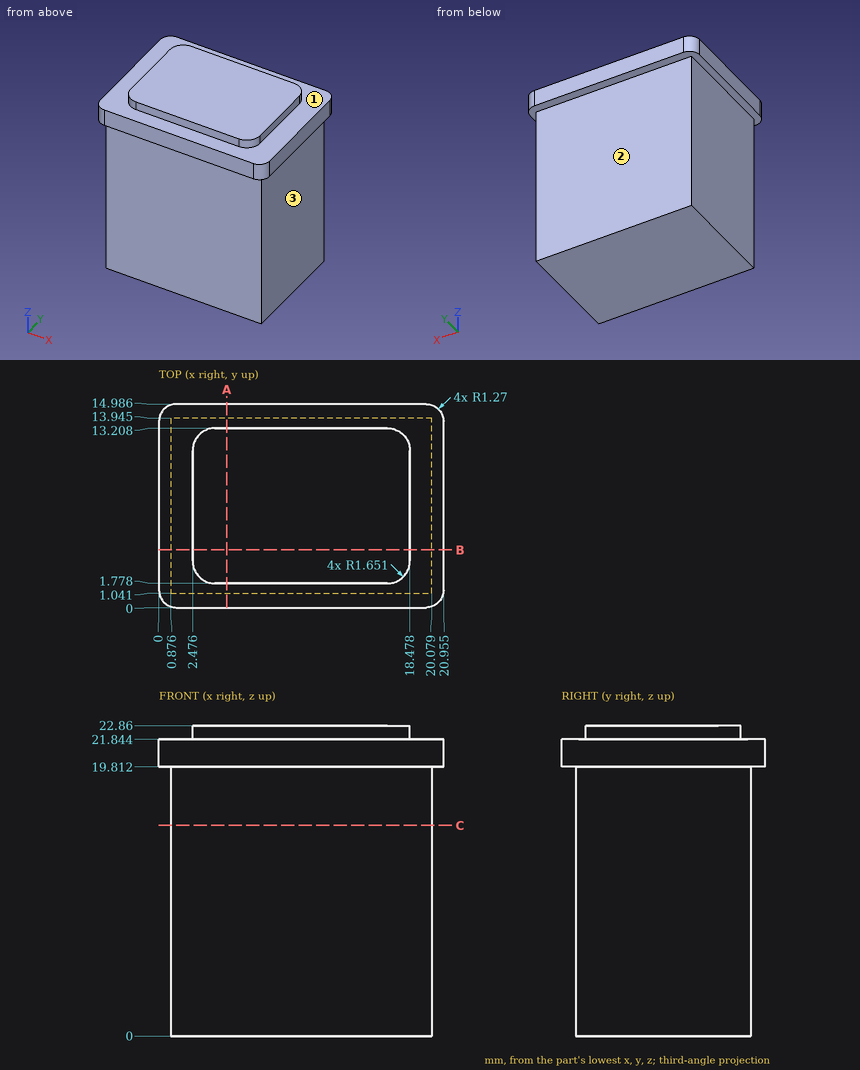
Geometry: see drawing. Coordinates: mm, zero at the bounding-box minimum. A direction names the side the tool comes from. Round coordinates to 2 decimals unless told otherwise and drop trailing zeros. Order: outer loops, then holes, each group sorted by start corner. A loop starts at its lowest first (then second) coordinate and runs counter-clockwise, first axis right, second up. Notation, with made-up numbers: (26.25, 56) - (44.25, 56) arc R12 ccw to (44.25, 72) - close; hole circle Ø1 at (-22.75, 42.5). An arc over 180 degrees is marked (long way). One line per question, with ' | ' between items. Start each with the question number.
1) Cut plane A-A, the plane x = 5. Return the cut outline in (y, z) (1 decimal), then the cut area to 3 significant figures.
2) Ray query, probe 1 along X at (y, z) = (9.25, 18); probe 2 along Y at (x, z) = (17.25, 17.5) (1 decimal); probe 3 along Z at (x, y) = (19, 1.25) (1 decimal). Return the intervals inside material, ascending.
3) Contact query for flat-ended pins moving along their axis: P1, Ø9.5, axis at x = 13, z = 7.5, coming from the -Y side; P2, Ø6, axis at x = 11.5, z = 7.5, coming from the +Y side (1 decimal); P3, Ø0.5, axis at y = 7.5, z = 22.5, coming from the -X side; P4, Ø0.5, axis at y = 6, z = 22, coming from the +X side (1 decimal). Output: stop coordinate, or through.
4) Cut plane C-C, the plane z = 15.5. Return the cut outline in (x, y) (1 decimal).
5) Set-up query: the marked faces 1, 2 and 3. Return all of +Z, -Z, +X, -X, +Y, -Y with unobstructed straight access to the full face (end or side cutting, diameter ignored); none if empty.
6) Cut plane B-B, the plane y = 4.25. Return the cut outline in (x, z) (1 decimal).
Worked out:
1) outline: (0, 19.8) - (1, 19.8) - (1, 0) - (13.9, 0) - (13.9, 19.8) - (15, 19.8) - (15, 21.8) - (13.2, 21.8) - (13.2, 22.9) - (1.8, 22.9) - (1.8, 21.8) - (0, 21.8) - close | area: 298 mm^2
2) probe 1: x = 0.88 to 20.08 | probe 2: y = 1 to 13.9 | probe 3: z = 0 to 21.8
3) P1: stops at y = 1.04 | P2: stops at y = 13.9 | P3: stops at x = 2.48 | P4: stops at x = 21
4) outline: (0.9, 1) - (20.1, 1) - (20.1, 13.9) - (0.9, 13.9) - close
5) face 1: +Z | face 2: -Z, +X, -X, +Y | face 3: -Z, +X, +Y, -Y
6) outline: (0, 19.8) - (0.9, 19.8) - (0.9, 0) - (20.1, 0) - (20.1, 19.8) - (21, 19.8) - (21, 21.8) - (18.5, 21.8) - (18.5, 22.9) - (2.5, 22.9) - (2.5, 21.8) - (0, 21.8) - close
